```python
from build123d import *

# Parameters (mm, degrees)
CUT_EXTRUDE1_DEPTH = 7.7


with BuildPart() as part:
    # Sketch1 → Revolve1 (revolve)
    with BuildSketch(Plane(origin=(0, 0, 0), x_dir=(0, 0, -1), z_dir=(1, 0, 0))):
        with BuildLine():
            Line((0, 0), (0, 6.85))
            Line((0, 6.85), (11.217157288, 6.85))
            Line((11.217157288, 6.85), (11.5, 6.567157288))
            Line((11.5, 6.567157288), (11.5, 5.9))
            Line((11.5, 5.9), (13.9, 5.9))
            Line((13.9, 5.9), (14, 5.8))
            Line((14, 5.8), (14.1, 5.9))
            Line((14.1, 5.9), (14.8, 5.9))
            Line((14.8, 5.9), (15, 5.7))
            Line((15, 5.7), (15, 4.669))
            Line((15, 4.669), (15.525, 4.669))
            ThreePointArc((15.525, 4.669), (15.790165043, 4.778834957), (15.9, 5.044))
            Line((15.9, 5.044), (15.9, 6.9))
            Line((15.9, 6.9), (17.268263788, 6.9))
            ThreePointArc((17.268263788, 6.9), (17.396821309, 6.853208889), (17.465225338, 6.734729636))
            Line((17.465225338, 6.734729636), (17.9, 4.269))
            Line((17.9, 4.269), (17.9, 0))
            Line((17.9, 0), (0, 0))
        make_face()
    revolve(axis=Axis((0, 0, -17.9), (0, 0, 1)))

    # Sketch2 → Revolve2 (revolve)
    with BuildSketch(Plane(origin=(0, 0, 0), x_dir=(0, 0, -1), z_dir=(1, 0, 0))):
        Polygon((-8, 0), (-8, 4.158121832), (-6.93615215, 4.772334675), (0, 4.988878168), (0, 0), align=None)
    revolve(axis=Axis((0, 0, 0), (0, 0, 1)))

    # Sketch3 → Cut-Revolve1 (revolve, cut)
    with BuildSketch(Plane(origin=(0, 0, 0), x_dir=(0, 0, -1), z_dir=(1, 0, 0))):
        Polygon((0, 6.85), (0, 5.05), (3.4, 5.05), (3.4, 6.65), (3.6, 6.85), align=None)
    revolve(axis=Axis((0, 0, -50), (0, 0, 1)), mode=Mode.SUBTRACT)

    # Sketch4 → Cut-Revolve2 (revolve, cut)
    with BuildSketch(Plane(origin=(0, 0, 0), x_dir=(0, 0, -1), z_dir=(1, 0, 0))):
        with BuildLine():
            Line((-8, 0), (-8, 3.1))
            Line((-8, 3.1), (-7.5, 2.6))
            Line((-7.5, 2.6), (-0.3, 2.6))
            Line((-0.3, 2.6), (-0.3, 3.969))
            Line((-0.3, 3.969), (17.6, 3.969))
            ThreePointArc((17.6, 3.969), (17.812132034, 4.056867966), (17.9, 4.269))
            Line((17.9, 4.269), (17.9, 0))
            Line((17.9, 0), (-8, 0))
        make_face()
    revolve(axis=Axis((0, 0, -17.9), (0, 0, 1)), mode=Mode.SUBTRACT)

    # Sketch5 → Cut-Extrude1 (cut)
    with BuildSketch(Plane.XY.offset(0.3)):
        Polygon((-2.5, -1.443375673), (0, -2.886751346), (2.5, -1.443375673), (2.5, 1.443375673), (0, 2.886751346), (-2.5, 1.443375673), align=None)
    extrude(amount=CUT_EXTRUDE1_DEPTH, mode=Mode.SUBTRACT)


solid = part.part
```
Check sheet for the modelled part. Datum: model origin and axes. Units: mm. A direction names the side the tool comes from. Round coordinates to 2 decimals unless told otherwise and drop trailing zeros. Write each loop counter-clockwise with the first axis right and the second up, starting at its lowest first coordinate (ties: lowest second). Pieces come first, ordered by that corner, then holes. Notation, with made-up numbers: (-2.75, 11) -> (31.25, 11) arc R24 ccw to (31.25, 28) -> close; hole circle Ø11 at (-29.75, 5.25). An arc over 180 degrees is marked (long way). Put each result on its own line as item: value.
(1) Sectioned sample at D-D (z = -7.5). Enter the section's corners in (x, y).
Values found:
outline: circle Ø13.7 at (0, 0); hole circle Ø7.94 at (0, 0)
(2) Material ranges on line 1 (Y direction, x = 0, z = -9.5); line 2 (X direction, y = 0, z = -11.75), recorded low to high.
Values found:
line 1: y = -6.85 to -3.97, 3.97 to 6.85
line 2: x = -5.9 to -3.97, 3.97 to 5.9
(3) Mould release check, pull along Z, two halves, no side actions. Record for faces 1 (the face through (-2, 5, -3.4)), 2 (the face through (1, -3, 0.3)), 3 (the face through (-1, -6, -11.5)): released by +Z, released by -Z, zero draft, split by the parting line, or undercut.
Values found:
face 1: released by +Z
face 2: released by -Z
face 3: undercut
(4) Tool access check on faces 4 (the face through (2.841, -3.705, -15.266)), 5 (the face through (1.291, -2.257, 3.85)), 6 (the face through (-1.517, 4.817, -1.724)). Record the directions out of +Z, -Z, +X, -X, +Y, -Y that give a thin tool (end or side, any length) a straight path to the whole face; none if there is none.
Values found:
face 4: none
face 5: +Z, -Z
face 6: +Z
(5) Sectioned sample at C-C (z = -12). Enter the section's corners in (x, y).
Values found:
outline: circle Ø11.8 at (0, 0); hole circle Ø7.94 at (0, 0)
(6) Sectioned sample at A-A (z = 1). Enter the section's corners in (x, y).
Values found:
outline: circle Ø9.92 at (0, 0); hole (-2.5, -1.44) -> (-1.87, -1.81) arc R2.6 ccw to (-0.63, -2.52) -> (0, -2.89) -> (0.63, -2.52) arc R2.6 ccw to (1.87, -1.81) -> (2.5, -1.44) -> (2.5, -0.71) arc R2.6 ccw to (2.5, 0.71) -> (2.5, 1.44) -> (1.87, 1.81) arc R2.6 ccw to (0.63, 2.52) -> (0, 2.89) -> (-0.63, 2.52) arc R2.6 ccw to (-1.87, 1.81) -> (-2.5, 1.44) -> (-2.5, 0.71) arc R2.6 ccw to (-2.5, -0.71) -> close
(7) Go/stop test with flat-tipped pins: pin 1 Ø5 at (y, z) = (4.5, -10.5) entering from -X; pin 2 Ø8 at (y, z) = (1, -1) entering from -X; pin 3 Ø4 at (y, z) = (4.5, -9.5) entering from +X. Record where each tip stops, or that it passes through.
Values found:
pin 1: stops at x = -6.55
pin 2: stops at x = -6.85
pin 3: stops at x = 6.38
(8) Sectioned sample at B-B (z = 4.75). Enter the section's corners in (x, y), plus the area to 3 significant figures.
Values found:
outline: circle Ø9.68 at (0, 0); hole (-2.5, -1.44) -> (-1.87, -1.81) arc R2.6 ccw to (-0.63, -2.52) -> (0, -2.89) -> (0.63, -2.52) arc R2.6 ccw to (1.87, -1.81) -> (2.5, -1.44) -> (2.5, -0.71) arc R2.6 ccw to (2.5, 0.71) -> (2.5, 1.44) -> (1.87, 1.81) arc R2.6 ccw to (0.63, 2.52) -> (0, 2.89) -> (-0.63, 2.52) arc R2.6 ccw to (-1.87, 1.81) -> (-2.5, 1.44) -> (-2.5, 0.71) arc R2.6 ccw to (-2.5, -0.71) -> close
area: 51.4 mm^2
